Check sheet for the drawn part. Datum: minimum x, y, z corner. Units: mm. Coordinates: 2 decimals unless noted, no trailing zeros. Write each loop counter-clockwise with the first axis right and the second up, starting at its lowest first coordinate (ties: lowest second). Pieces come first, ordered by that corner, then holes. Notation, with made-up numbers: (-25, 62.5) - (1, 62.5) arc R33 cw to (1, 91.5) - close; hole circle Ø7 at (12.5, 42). An arc over 180 degrees is marked (long way). Write each question's results on one line, items separated by ' | '.
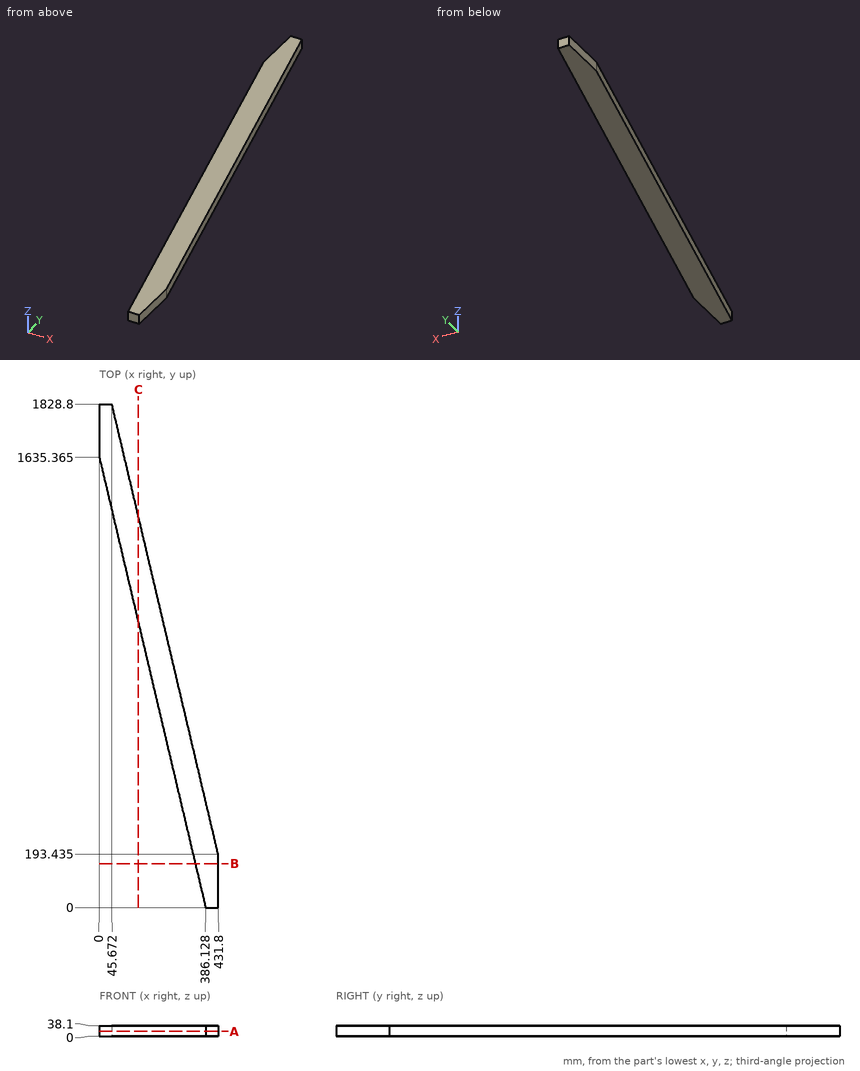
1. Sectioned sample at B-B (y = 159.5). Record the cut outline in (x, z).
Values follow:
outline: (348.47, 0) - (431.8, 0) - (431.8, 38.1) - (348.47, 38.1) - close
2. Sectioned sample at C-C (x = 142). Record the cut outline in (y, z), then the cut area to 3 significant figures.
Values follow:
outline: (1033.95, 0) - (1420.82, 0) - (1420.82, 38.1) - (1033.95, 38.1) - close | area: 14,700 mm^2
3. Material ranges on L1, parallel to X at y = 1753, z = 6; L2, parallel to X at y = 963.5, z = 19.5 (1 decimal), recorded low to high. Write a range as [from, to].
Values follow:
L1: x = [0, 63.57] | L2: x = [158.6, 250]
4. Go/stop test with flat-tipped pins: pin 1 (8 mm diameter, centred on y = 403, z = 8, fed in from -X); pin 2 (1.5 mm diameter, centred on y = 547.5, z = 21, fed in from -X); pin 3 (1 mm diameter, centred on y = 1479, z = 30.5, fed in from +X). Record where each tip stops, or that it passes through.
Values follow:
pin 1: stops at x = 290.03 | pin 2: stops at x = 256.68 | pin 3: stops at x = 128.38
5. Sectioned sample at A-A (z = 17). Record the cut outline in (x, y) (1 decimal).
Values follow:
outline: (0, 1635.4) - (386.1, 0) - (431.8, 0) - (431.8, 193.4) - (45.7, 1828.8) - (0, 1828.8) - close
